The figure shows three views and two pictorial views of one solid part (mm, origin at its lowest corner). Answer the questions. Round coordinates to 2 decimals unless told otherwise and drop trailing zeros. Order: outer loops, then holes, each group sorted by start corner. A loop starts at its lowest first (then second) coordinate and runs counter-clockwise, first axis right, second up. Notation, with made-up numbers: (23.25, 73) -> (32.25, 73) arc R22 cw to (32.25, 111) -> close; hole circle Ø11 at (41.5, 61.5). An arc over 180 degrees is marked (long way). Answer in a Markdown table with one row per item. Add a question column.
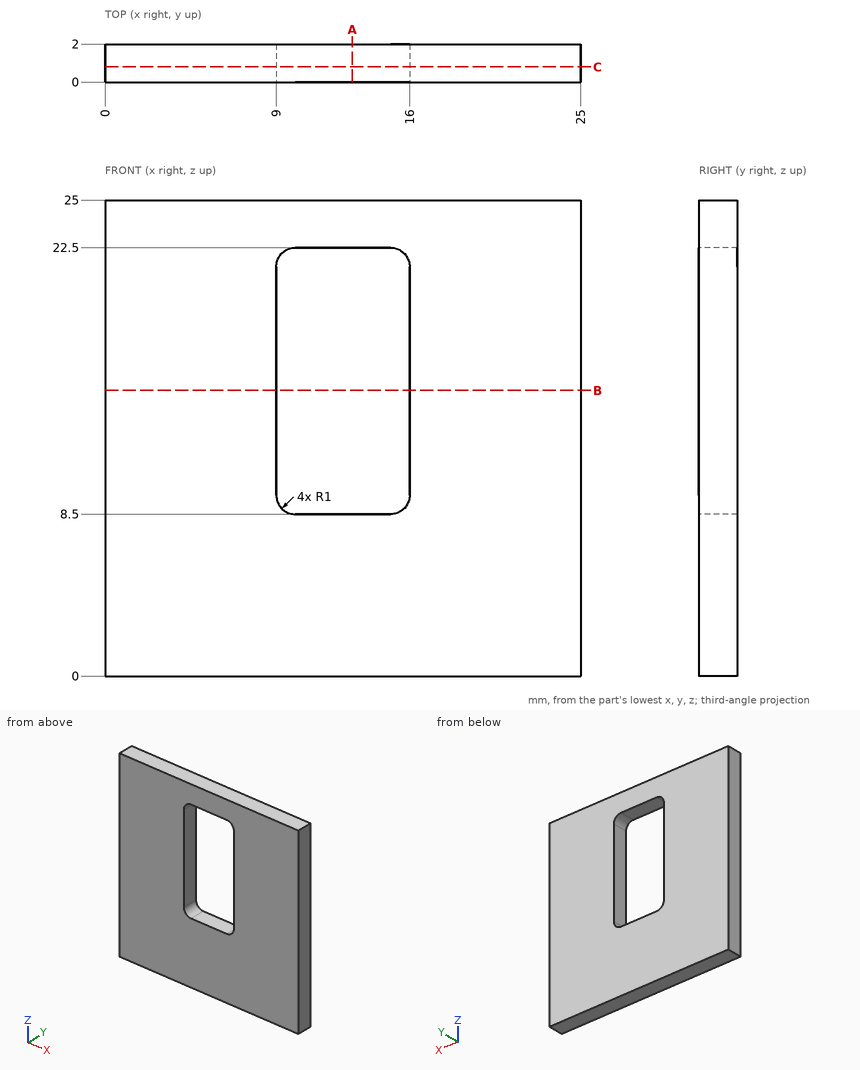
1. The part is cut by section B-B (z = 15). Give the vertices of the cut face in (x, y), then the cut area to 3 significant figures.
2. Straight lines are drawn through the part: line 1 along Z through (x, y) = (14.5, 1.15); line 2 along X through (y, z) = (0.4, 19.5); line 3 along Z through (x, y) = (9.25, 1). For each, find the intervals that lie inside material, in ascending order.
3. The part is cut by section C-C (y = 0.8). Give the vertices of the cut face in (x, z).
4. The part is cut by section A-A (x = 13). Give the vertices of the cut face in (y, z).
Report:
| question | item | result |
|---|---|---|
| 1 | outline | (0, 0) -> (9, 0) -> (9, 2) -> (0, 2) -> close; (16, 0) -> (25, 0) -> (25, 2) -> (16, 2) -> close |
| 1 | area | 36.0 mm^2 |
| 2 | line 1 | z = 0 to 8.5, 22.5 to 25 |
| 2 | line 2 | x = 0 to 9, 16 to 25 |
| 2 | line 3 | z = 0 to 8.84, 22.16 to 25 |
| 3 | outline | (0, 0) -> (25, 0) -> (25, 25) -> (0, 25) -> close; hole (9, 9.5) arc R1 ccw to (10, 8.5) -> (15, 8.5) arc R1 ccw to (16, 9.5) -> (16, 21.5) arc R1 ccw to (15, 22.5) -> (10, 22.5) arc R1 ccw to (9, 21.5) -> close |
| 4 | outline | (0, 0) -> (2, 0) -> (2, 8.5) -> (0, 8.5) -> close; (0, 22.5) -> (2, 22.5) -> (2, 25) -> (0, 25) -> close |
